```python
from build123d import *

# Parameters (mm, degrees)
F1_W     = 23
F1_H     = 15
F2_DEPTH = 10
F4_DEPTH = 7
F5_R     = 2
F6_R     = 3.7
F6_R_2   = 1.7
F7_DEPTH = 7
F8_DEPTH = 25


with BuildPart() as f2:
    # F1 (on Top) → F2 (new body)
    with BuildSketch(Plane.XY):
        with Locations((1.8, 0)):
            Rectangle(F1_W, F1_H)
    extrude(amount=F2_DEPTH)

    # F3 (on face) → F4 (cut)
    with BuildSketch(Plane.XY.offset(10)):
        with BuildLine():
            ThreePointArc((5.5722526863, -1.2), (5.6679731965, -0.6033902916), (5.7, 0))
            ThreePointArc((5.7, 0), (5.6679731965, 0.6033902916), (5.5722526863, 1.2))
            Line((5.5722526863, 1.2), (1.572670415, 1.2))
            Line((1.572670415, 1.2), (1.572670415, -1.2))
            Line((1.572670415, -1.2), (5.5722526863, -1.2))
        make_face()
        with BuildLine():
            ThreePointArc((5.5722526863, 1.2), (5.6679731965, 0.6033902916), (5.7, 0))
            ThreePointArc((5.7, 0), (5.6679731965, -0.6033902916), (5.5722526863, -1.2))
            Line((5.5722526863, -1.2), (15.8343315125, -1.2))
            Line((15.8343315125, -1.2), (15.8343315125, 1.2))
            Line((15.8343315125, 1.2), (5.5722526863, 1.2))
        make_face()
        with BuildLine():
            Line((1.572670415, 1.2), (5.5722526863, 1.2))
            ThreePointArc((5.5722526863, 1.2), (-5.7, 0), (5.5722526863, -1.2))
            Line((5.5722526863, -1.2), (1.572670415, -1.2))
            Line((1.572670415, -1.2), (1.572670415, 1.2))
        make_face()
    extrude(amount=-F4_DEPTH, mode=Mode.SUBTRACT)

    # F5
    f5_edges = [f2.edges().sort_by_distance(p)[0] for p in [
        (5.572253, 1.2, 6.5),
        (5.572253, -1.2, 6.5),
    ]]
    fillet(f5_edges, radius=F5_R)

    # F6 (on face) → F7 (join)
    with BuildSketch(Plane.XY.offset(3)):
        Circle(F6_R)
        Circle(F6_R_2, mode=Mode.SUBTRACT)
    extrude(amount=F7_DEPTH)

    # F8 (cut): a face of the model
    f8_faces = [f2.faces().sort_by_distance(p)[0] for p in [
        (0, 0, 3),
    ]]
    extrude(f8_faces, amount=-F8_DEPTH, mode=Mode.SUBTRACT)


solid = f2.part
```
Check sheet for the modelled part. Datum: model origin and axes. Units: mm. A direction names the side the tool comes from. Coordinates: 2 decimals unless noted, no trailing zeros. Order: outer loops, then holes, each group sorted by start corner. A loop starts at its lowest first (then second) coordinate and runs counter-clockwise, first axis right, second up. Notation, with made-up numbers: M 57,89.5 L 98,89.5 A14 ccw 98,106.5 Z; hole C 44,9 d10. An arc over 180 degrees is marked long. Write each question's results on one line, items separated by ' | '. Start each with the question number.
1. Mould release check, pull along X, two halves, no side actions. Record for faces 1 (the face through (-9.7, 0, 5)), 2 (the face through (13.3, -2, 5)), 3 (the face through (4, -1, 3)): +X half, -X half, draft (parallel to the pull), parting line (faces both ways), or undercut.
2. Cross-section at C-C on y = 0. Record the cut outline in (x, z), and give its area (3 significant figures).
3. Cross-section at B-B on x = 0. Record the cut outline in (y, z).
4. Cross-section at A-A on z = 5.25. Record the cut outline in (x, y), and give its area (3 significant figures).
5. Cross-section at D-D on x = 6.5. Record the cut outline in (y, z).
6. Go/stop test with a flat-tipped pin: P1, Ø9, axis at x = 0, y = 0, coming from the +Z side. Record where the tip stops, or that it passes through.
7. Material ranges on probe 1 along Y at (x, z) = (0, 5.25); probe 2 along X at (y, z) = (-2.5, 5); probe 3 along X at (y, z) = (1.75, 5.25), recorded low to high.
8. Access from +Z, -Z, +X, -X, +Y, -Y to the whole of each face (thin tool, end or side, straight path). Record for faces 4 (the face through (1, -2, 10)), 5 (the face through (10, 1.2, 7)), 6 (the face through (-5.696, 0.216, 6.549)).
Checks:
1) face 1: -X half | face 2: +X half | face 3: undercut
2) outline: M -9.7,0 L -1.7,0 L -1.7,10 L -3.7,10 L -3.7,3 L -5.7,3 L -5.7,10 L -9.7,10 Z; M 1.7,0 L 13.3,0 L 13.3,3 L 3.7,3 L 3.7,10 L 1.7,10 Z | area: 115 mm²
3) outline: M -7.5,0 L -1.7,0 L -1.7,10 L -3.7,10 L -3.7,3 L -5.7,3 L -5.7,10 L -7.5,10 Z; M 1.7,0 L 7.5,0 L 7.5,10 L 5.7,10 L 5.7,3 L 3.7,3 L 3.7,10 L 1.7,10 Z
4) outline: M -9.7,-7.5 L 13.3,-7.5 L 13.3,-1.2 L 7,-1.2 A2 ccw 5.18,-2.37 A5.7 cw long 5.18,2.37 A2 ccw 7,1.2 L 13.3,1.2 L 13.3,7.5 L -9.7,7.5 Z; C 0,0 d7.4; hole C 0,0 d3.4 | area: 258 mm²
5) outline: M -7.5,0 L 7.5,0 L 7.5,10 L 1.26,10 L 1.26,3 L -1.26,3 L -1.26,10 L -7.5,10 Z
6) P1: stops at z = 10
7) probe 1: y = -7.5 to -5.7, -3.7 to -1.7, 1.7 to 3.7, 5.7 to 7.5 | probe 2: x = -9.7 to -5.12, -2.73 to 2.73, 5.12 to 13.3 | probe 3: x = -9.7 to -5.42, -3.26 to 3.26, 5.63 to 13.3
8) face 4: +Z, +X, -X, +Y, -Y | face 5: +Z, +X | face 6: +Z
